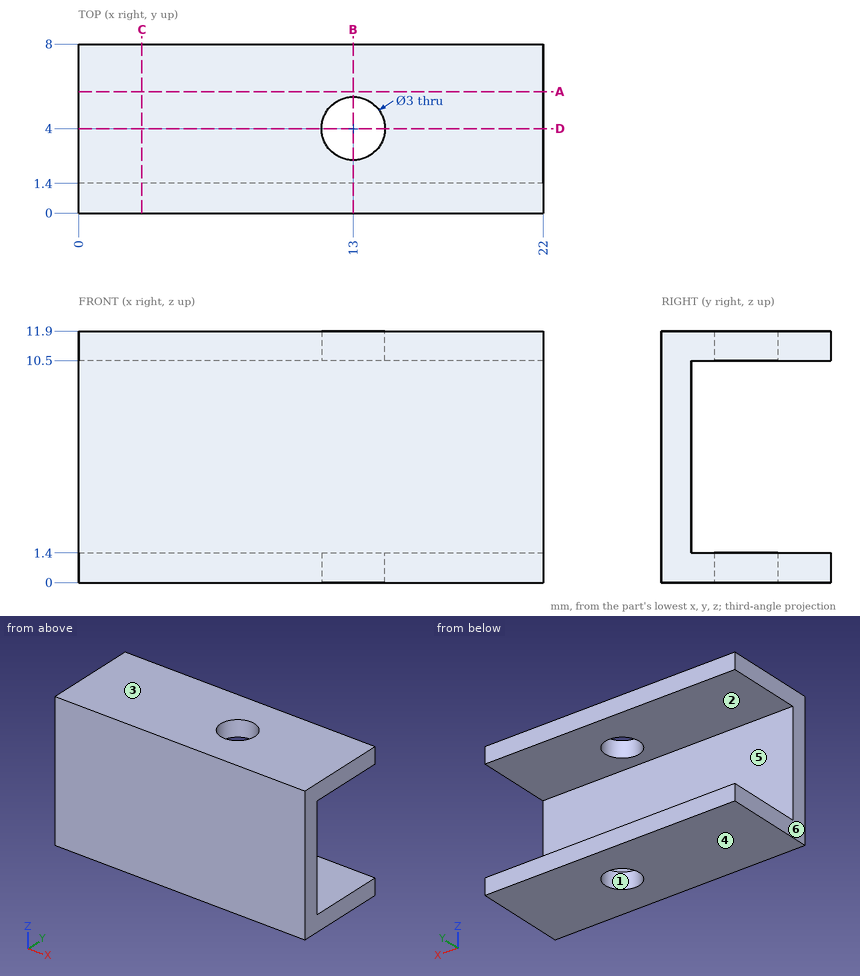
Input: dimensioned drawing with shaded views. Units: mm. Origin: part minimum x, y, z. A direction names the side the tool comes from. Give positions to 0.01 mm unless a question says otherwise; leave off trailing zeros. Order: outer loops, then holes, each group sorted by start corner. A loop starts at its lowest first (then second) coordinate and runs counter-clockwise, first axis right, second up.
(1) Section query D-D (y = 4). Return the cut outline in (x, z), plus the area to 3 significant figures.
(2) Section query B-B (x = 13). Return the cut outline in (y, z).
(3) Pull-direction query (Z, two-part tool) for the marked faces 3, 4, 5 and 6; classes: +Z half, -Z half, draft (parallel to the pull), parting line (faces both ways), or undercut.
(4) Section query A-A (y = 5.75). Return the cut outline in (x, z).
(5) Section query C-C (x = 3). Return the cut outline in (y, z), plus the area to 3 significant figures.
(6) Access query for the marked faces 1 and 2. Directions: +Z, -Z, +X, -X, +Y, -Y. A direction counts if a zero-diameter tool reaches every point of the face in a straight line with its end or side. Return the directions, or none.
(7) Contact query for a flat-ended pin moving along its axis: P1, Ø3, axis at y = 3, z = 3, coming from the -X side. Output: stop coordinate, or through.
(8) Material intervals for line 1 along X through (y, z) = (4, 11); line 2 along Y through (x, z) = (13, 11); line 3 along Z through (x, y) = (3.5, 7.5), sorted ascending.
Outcome:
1. outline: (0, 0) - (11.5, 0) - (11.5, 1.4) - (0, 1.4) - close; (0, 10.5) - (11.5, 10.5) - (11.5, 11.9) - (0, 11.9) - close; (14.5, 0) - (22, 0) - (22, 1.4) - (14.5, 1.4) - close; (14.5, 10.5) - (22, 10.5) - (22, 11.9) - (14.5, 11.9) - close
1. area: 53.2 mm2
2. outline: (0, 0) - (2.5, 0) - (2.5, 1.4) - (1.4, 1.4) - (1.4, 10.5) - (2.5, 10.5) - (2.5, 11.9) - (0, 11.9) - close; (5.5, 0) - (8, 0) - (8, 1.4) - (5.5, 1.4) - close; (5.5, 10.5) - (8, 10.5) - (8, 11.9) - (5.5, 11.9) - close
3. face 3: +Z half
3. face 4: -Z half
3. face 5: undercut
3. face 6: draft
4. outline: (0, 0) - (22, 0) - (22, 1.4) - (0, 1.4) - close; (0, 10.5) - (22, 10.5) - (22, 11.9) - (0, 11.9) - close
5. outline: (0, 0) - (8, 0) - (8, 1.4) - (1.4, 1.4) - (1.4, 10.5) - (8, 10.5) - (8, 11.9) - (0, 11.9) - close
5. area: 35.1 mm2
6. face 1: +Z, -Z
6. face 2: +X, -X, +Y
7. P1: passes through
8. line 1: x = 0 to 11.5, 14.5 to 22
8. line 2: y = 0 to 2.5, 5.5 to 8
8. line 3: z = 0 to 1.4, 10.5 to 11.9
